The drawing under review shows one solid part. Ordinate dimensions are in mm from its lowest x, y, z. Give positions to 0.01 mm unless a question says otherwise; leave off trailing zeros. Order: outer loops, then holes, each group sorted by start corner. A loop starts at its lowest first (then second) coordinate and runs counter-clockwise, first axis right, second up. Notation, with made-up numbers: (62, 77.5) -> (82, 77.5) arc R27 ccw to (82, 105.5) -> close; hole circle Ø8 at (-10.5, 23). An arc over 180 degrees is marked (long way). Use CSV: the item, a comma, the result in double quotes. Start each with the question number.
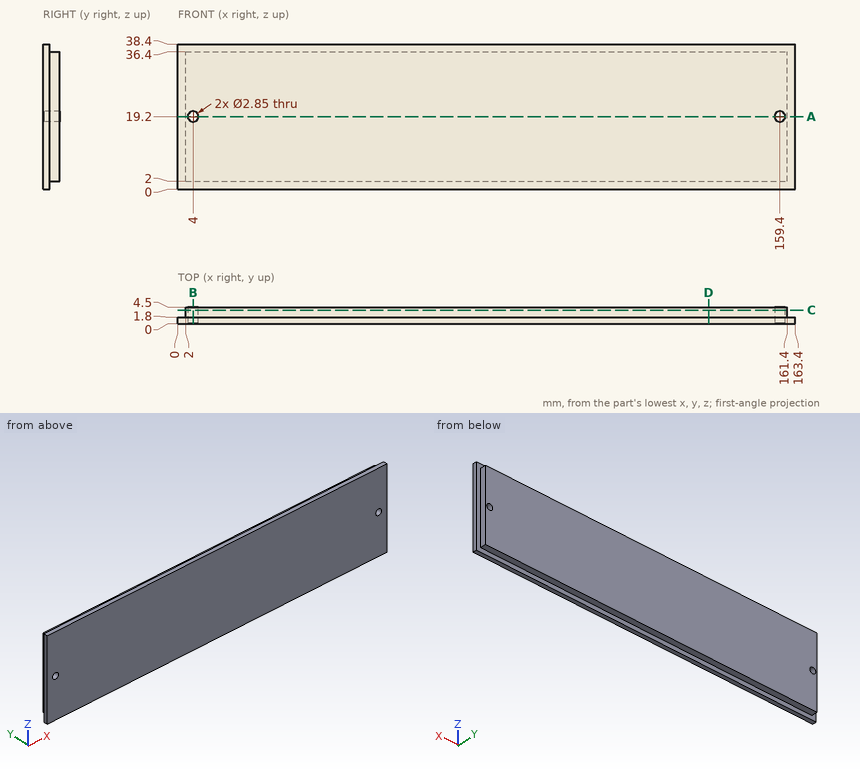
1. Consider section D-D (x = 140.5). State the section outline as (y, z) points.
2. Consider section C-C (y = 3.65). State the section outline as (x, z) points (3 decimals).
3. To check wall thickness, follow L1, parallel to Z at x = 4, y = 2.2 (3 decimals); L2, parallel to Z at x = 159.4, y = 1.25 (3 decimals); L3, parallel to Z at x = 9.5, y = 2.85. State the ranges of each line that lie inside material, in increasing order. Write a range as [from, to].
4. Consider section B-B (x = 4). State the section outline as (y, z) points (3 decimals), plus the area to 3 significant figures.
5. Clearance check with flat-ended pins moving along their axes: P1, Ø0.8, axis at y = 3.5, z = 15.5, coming from the -X side; P2, Ø2, axis at x = 111.5, y = 3.5, coming from the -Z side. State where each tip first meets the part, or that it passes through.
6. Consider section A-A (z = 19.2). State the section outline as (x, y) points (3 decimals).
Answer list:
1,outline,"(0, 0) -> (1.8, 0) -> (1.8, 2) -> (4.5, 2) -> (4.5, 36.4) -> (1.8, 36.4) -> (1.8, 38.4) -> (0, 38.4) -> close"
2,outline,"(2, 2) -> (161.4, 2) -> (161.4, 36.4) -> (2, 36.4) -> close; hole circle Ø2.85 at (4, 19.2); hole circle Ø2.85 at (159.4, 19.2)"
3,L1,"[2, 17.775], [20.625, 36.4]"
3,L2,"[0, 17.775], [20.625, 38.4]"
3,L3,"[2, 36.4]"
4,outline,"(0, 0) -> (1.8, 0) -> (1.8, 2) -> (4.5, 2) -> (4.5, 17.775) -> (0, 17.775) -> close; (0, 20.625) -> (4.5, 20.625) -> (4.5, 36.4) -> (1.8, 36.4) -> (1.8, 38.4) -> (0, 38.4) -> close"
4,area,"149 mm2"
5,P1,"x = 2"
5,P2,"z = 2"
6,outline,"(0, 0) -> (2.575, 0) -> (2.575, 4.5) -> (2, 4.5) -> (2, 1.8) -> (0, 1.8) -> close; (5.425, 0) -> (157.975, 0) -> (157.975, 4.5) -> (5.425, 4.5) -> close; (160.825, 0) -> (163.4, 0) -> (163.4, 1.8) -> (161.4, 1.8) -> (161.4, 4.5) -> (160.825, 4.5) -> close"
